Work out the finished part from the listing and answer in its coordinate system (mm). Coordinates: 2 decimals unless noted, no trailing zeros. Loops run counter-clockwise (first coordinate to the right, second up) from the corner with the lowest first, then second, coordinate; pieces in that order, holes last.
```python
from build123d import *

# Parameters (mm, degrees)
SKETCH1_R           = 2.5
BOSS_EXTRUDE1_DEPTH = 1
SKETCH2_W           = 100
SKETCH2_H           = 21
SKETCH2_R           = 2.5
BOSS_EXTRUDE2_DEPTH = 1
SKETCH3_W           = 101
SKETCH3_H           = 21
SKETCH3_R           = 2.5
BOSS_EXTRUDE5_DEPTH = 1


with BuildPart() as part:
    # Sketch1 → Boss-Extrude1 (new body)
    with BuildSketch(Plane(origin=(0, 0, 0), x_dir=(1, 0, 0), z_dir=(0, 1, 0))):
        Polygon((0, 0), (0, -100), (100, -100), (100, -60), (40, 0), align=None)
        with Locations((10, -5)):
            Circle(SKETCH1_R, mode=Mode.SUBTRACT)
        with Locations((30, -5)):
            Circle(SKETCH1_R, mode=Mode.SUBTRACT)
        with Locations((30, -55)):
            Circle(SKETCH1_R, mode=Mode.SUBTRACT)
        with Locations((10, -55)):
            Circle(SKETCH1_R, mode=Mode.SUBTRACT)
        with Locations((30, -30)):
            Circle(SKETCH1_R, mode=Mode.SUBTRACT)
        with Locations((10, -30)):
            Circle(SKETCH1_R, mode=Mode.SUBTRACT)
        with Locations((50, -70)):
            Circle(SKETCH1_R, mode=Mode.SUBTRACT)
        with Locations((50, -90)):
            Circle(SKETCH1_R, mode=Mode.SUBTRACT)
        with Locations((95, -70)):
            Circle(SKETCH1_R, mode=Mode.SUBTRACT)
        with Locations((95, -90)):
            Circle(SKETCH1_R, mode=Mode.SUBTRACT)
        with Locations((5, -70)):
            Circle(SKETCH1_R, mode=Mode.SUBTRACT)
        with Locations((5, -90)):
            Circle(SKETCH1_R, mode=Mode.SUBTRACT)
    extrude(amount=BOSS_EXTRUDE1_DEPTH)

    # Sketch2 → Boss-Extrude2 (add)
    with BuildSketch(Plane.ZY):
        with Locations((50, -9.5)):
            Rectangle(SKETCH2_W, SKETCH2_H)
        with Locations((5, -10)):
            Circle(SKETCH2_R, mode=Mode.SUBTRACT)
        with Locations((15, -10)):
            Circle(SKETCH2_R, mode=Mode.SUBTRACT)
        with Locations((25, -10)):
            Circle(SKETCH2_R, mode=Mode.SUBTRACT)
        with Locations((35, -10)):
            Circle(SKETCH2_R, mode=Mode.SUBTRACT)
        with Locations((45, -10)):
            Circle(SKETCH2_R, mode=Mode.SUBTRACT)
        with Locations((55, -10)):
            Circle(SKETCH2_R, mode=Mode.SUBTRACT)
        with Locations((65, -10)):
            Circle(SKETCH2_R, mode=Mode.SUBTRACT)
        with Locations((75, -10)):
            Circle(SKETCH2_R, mode=Mode.SUBTRACT)
    extrude(amount=BOSS_EXTRUDE2_DEPTH)

    # Sketch3 → Boss-Extrude5 (add)
    with BuildSketch(Plane.XY.offset(100)):
        with Locations((49.5, -9.5)):
            Rectangle(SKETCH3_W, SKETCH3_H)
        with Locations((95, -9.5)):
            Circle(SKETCH3_R, mode=Mode.SUBTRACT)
        with Locations((85, -9.5)):
            Circle(SKETCH3_R, mode=Mode.SUBTRACT)
        with Locations((75, -9.5)):
            Circle(SKETCH3_R, mode=Mode.SUBTRACT)
        with Locations((65, -9.5)):
            Circle(SKETCH3_R, mode=Mode.SUBTRACT)
        with Locations((55, -9.5)):
            Circle(SKETCH3_R, mode=Mode.SUBTRACT)
        with Locations((45, -9.5)):
            Circle(SKETCH3_R, mode=Mode.SUBTRACT)
        with Locations((35, -9.5)):
            Circle(SKETCH3_R, mode=Mode.SUBTRACT)
        with Locations((25, -9.5)):
            Circle(SKETCH3_R, mode=Mode.SUBTRACT)
        with Locations((15, -9.5)):
            Circle(SKETCH3_R, mode=Mode.SUBTRACT)
        with Locations((5, -9.5)):
            Circle(SKETCH3_R, mode=Mode.SUBTRACT)
    extrude(amount=BOSS_EXTRUDE5_DEPTH)


solid = part.part
```
1. A cutting plane is placed at A-A, the plane z = 25. Give the vertices of the cut face in (x, y).
2. Straight lines are drawn through the part: probe 1 along Z at (x, y) = (5, 0.3); probe 2 along Y at (x, z) = (55, 100.6); probe 3 along X at (y, z) = (0.3, 30). For each, find the intervals that lie inside material, in ascending order.
3. Each of these flat-tipped pins is pushed along its axis until it touches: P1, Ø3, axis at y = -16, z = 58, coming from the +X side; P2, Ø1, axis at x = 25, z = 52, coming from the -Y side; P3, Ø6.5, axis at y = -10, z = 25, coming from the -X side; P4, Ø8, axis at x = 75, y = -9.5, coming from the -Z side. Where does it stop, or does it pass through?
4. A cutting plane is placed at C-C, the plane z = 70. Give the vertices of the cut face in (x, y).
5. A cutting plane is placed at B-B, the plane x = 15. Give the vertices of the cut face in (y, z).
6. Determine the mould class of faces 1 (the cylindrical face through (-0.49, -12.22, 66.15)), 2 (the flat face through (10.5, 0.6, 0)), 3 (the cylindrical face through (66.15, -11.72, 100.49)) for opening direction Z: released by +Z, released by -Z, zero draft, split by the parting line, or undercut.
7. A cutting plane is placed at D-D, the plane x = 95. Give the vertices of the cut face in (y, z).
Answers below:
1. outline: (-1, -20) - (0, -20) - (0, -12.5) - (-1, -12.5) - close; (-1, -7.5) - (0, -7.5) - (0, 0) - (65, 0) - (65, 1) - (-1, 1) - close
2. probe 1: z = 0 to 67.5, 72.5 to 87.5, 92.5 to 101
2. probe 2: y = -20 to -12, -7 to 1
2. probe 3: x = -1 to 7.5, 12.5 to 27.5, 32.5 to 70
3. P1: stops at x = 0
3. P2: stops at y = 0
3. P3: stops at x = -1
3. P4: stops at z = 100
4. outline: (-1, -20) - (0, -20) - (0, 0) - (2.5, 0) - (2.5, 1) - (-1, 1) - close; (7.5, 0) - (47.5, 0) - (47.5, 1) - (7.5, 1) - close; (52.5, 0) - (92.5, 0) - (92.5, 1) - (52.5, 1) - close; (97.5, 0) - (100, 0) - (100, 1) - (97.5, 1) - close
5. outline: (-20, 100) - (-12, 100) - (-12, 101) - (-20, 101) - close; (-7, 100) - (0, 100) - (0, 0) - (1, 0) - (1, 101) - (-7, 101) - close
6. face 1: undercut
6. face 2: released by -Z
6. face 3: zero draft
7. outline: (-20, 100) - (-12, 100) - (-12, 101) - (-20, 101) - close; (-7, 100) - (0, 100) - (0, 92.5) - (1, 92.5) - (1, 101) - (-7, 101) - close; (0, 55) - (1, 55) - (1, 67.5) - (0, 67.5) - close; (0, 72.5) - (1, 72.5) - (1, 87.5) - (0, 87.5) - close
